```python
from build123d import *

# Parameters (mm, degrees)
F0_W      = 10
F0_H      = 30
F0_R      = 2.125
F1_DEPTH  = 5
F2_W      = 10
F2_H      = 30
F3_DEPTH  = 4
F4_W      = 10
F4_H      = 14.15
F5_DEPTH  = 20
F7_DEPTH  = 10.001
F8_R      = 2.125
F9_DEPTH  = 22.076
F11_DEPTH = 4


with BuildPart() as f1:
    # F0 (on Top) → F1 (new body)
    with BuildSketch(Plane.XY):
        Rectangle(F0_W, F0_H)
        with Locations((1, -10)):
            Circle(F0_R, mode=Mode.SUBTRACT)
        with Locations((1, 10)):
            Circle(F0_R, mode=Mode.SUBTRACT)
    extrude(amount=F1_DEPTH)

    # F2 (on face) → F3 (join)
    with BuildSketch(Plane.XY.offset(5)):
        Rectangle(F2_W, F2_H)
        Polygon((-0.68875, -7.075), (2.68875, -7.075), (4.377499, -10), (2.68875, -12.925), (-0.68875, -12.925), (-2.377499, -10), align=None, mode=Mode.SUBTRACT)
        Polygon((4.377499, 10), (2.68875, 7.075), (-0.68875, 7.075), (-2.377499, 10), (-0.68875, 12.925), (2.68875, 12.925), align=None, mode=Mode.SUBTRACT)
    extrude(amount=F3_DEPTH)

    # F4 (on face) → F5 (join)
    with BuildSketch(Plane.XY.offset(9)):
        Rectangle(F4_W, F4_H)
    extrude(amount=F5_DEPTH)

    # F6 (on face) → F7 (cut, through all)
    with BuildSketch(Plane.YZ.offset(5)):
        with BuildLine():
            ThreePointArc((-3, 12.139388), (0, 5), (3, 12.139388))
            Line((3, 12.139388), (3, 29))
            Line((3, 29), (-3, 29))
            Line((-3, 29), (-3, 12.139388))
        make_face()
    extrude(amount=-F7_DEPTH, mode=Mode.SUBTRACT)

    # F8 (on face) → F9 (cut, through all)
    with BuildSketch(Plane.XZ.offset(7.075)):
        with Locations((0, 21.5)):
            Circle(F8_R)
    extrude(amount=-F9_DEPTH, mode=Mode.SUBTRACT)

    # F10 (on face) → F11 (join)
    with BuildSketch(Plane(origin=(0, 7.075, 0), x_dir=(-1, 0, 0), z_dir=(0, 1, 0))):
        Polygon((5, 18.613249), (5, 24.386751), (0, 27.273503), (-5, 24.386751), (-5, 18.613249), (0, 15.726497), align=None)
        Polygon((0, 24.877499), (2.925, 23.18875), (2.925, 19.81125), (0, 18.122501), (-2.925, 19.81125), (-2.925, 23.18875), align=None, mode=Mode.SUBTRACT)
    extrude(amount=F11_DEPTH)


solid = f1.part
```
Verification items for the finished model (mm, model axes). A direction names the side the tool comes from. Coordinates: 2 decimals unless noted, no trailing zeros. Loops run counter-clockwise (first coordinate to the right, second up) from the corner with the lowest first, then second, coordinate; pieces in that order, holes last. Notation, with made-up numbers: (-14, 64.25) -> (31, 64.25) arc R28 cw to (31, 100.25) -> close; hole circle Ø4 at (37.5, -32.5). An arc over 180 degrees is marked (long way). Answer in a Markdown table with one row per item.
1) Draft check along Y on faces 5 (the face through (-1.521, -11.483, 6.972)), 6 (the face through (0, 7.075, 24)), 7 (the face through (-1, 13, 9)), 8 (the face through (-1.521, 8.517, 6.972)). Enter one of: released by +Y, released by -Y, zero draft, split by the parting line, or undercut.
The answers:
| item | result |
|---|---|
| face 5 | undercut |
| face 6 | released by +Y |
| face 7 | zero draft |
| face 8 | undercut |
2) Section check D-D (y = -7.5). Record the cut outline in (x, z).
The answers:
| item | result |
|---|---|
| outline | (-5, 0) -> (5, 0) -> (5, 9) -> (2.93, 9) -> (2.93, 5) -> (-0.93, 5) -> (-0.93, 9) -> (-5, 9) -> close |
3) Section check C-C (x = 1). Give the number of separate pieces and of enclosed holes in the cut face, and give its area (3 significant figures).
The answers:
| item | result |
|---|---|
| separate pieces | 5 |
| enclosed holes | 0 |
| area | 301 mm2 |
4) Section check A-A (z = 21.5). Record the cut outline in (x, y) (3 decimals).
The answers:
| item | result |
|---|---|
| outline | (-5, -7.075) -> (-2.125, -7.075) -> (-2.125, -3) -> (-5, -3) -> close; (-5, 3) -> (-2.125, 3) -> (-2.125, 7.075) -> (-2.925, 7.075) -> (-2.925, 11.075) -> (-5, 11.075) -> close; (2.125, -7.075) -> (5, -7.075) -> (5, -3) -> (2.125, -3) -> close; (2.125, 3) -> (5, 3) -> (5, 11.075) -> (2.925, 11.075) -> (2.925, 7.075) -> (2.125, 7.075) -> close |
5) Section check B-B (y = 9). Record the cut outline in (x, z) (1 decimal).
The answers:
| item | result |
|---|---|
| outline | (-5, 0) -> (-0.9, 0) -> (-0.9, 5) -> (-1.8, 5) -> (-1.8, 9) -> (-5, 9) -> close; (-5, 18.6) -> (0, 15.7) -> (5, 18.6) -> (5, 24.4) -> (0, 27.3) -> (-5, 24.4) -> close; (2.9, 0) -> (5, 0) -> (5, 9) -> (3.8, 9) -> (3.8, 5) -> (2.9, 5) -> close; hole (-2.9, 19.8) -> (0, 18.1) -> (2.9, 19.8) -> (2.9, 23.2) -> (0, 24.9) -> (-2.9, 23.2) -> close |
6) Access from +Z, -Z, +X, -X, +Y, -Y to the whole of each face (thin tool, end or side, straight path). Record for faces 1 (the face through (3.2, -9.3, 5)), 2 (the face through (2.535, 9.047, 17.19)), 3 (the face through (1.442, 9.047, 18.955)), 4 (the face through (0, 3, 19)).
The answers:
| item | result |
|---|---|
| face 1 | +Z |
| face 2 | +X, +Y |
| face 3 | +Y |
| face 4 | +Z, +X, -X |
7) Depth check by flat-ended pin: P1, Ø5.5, axis at x = 1, y = -10, coming from the +Z side; P2, Ø1.5, axis at x = -4, z = 25.5, coming from the -Y side (3 decimals); P3, Ø2, axis at x = 2, z = 11, coming from the +Y side (3 decimals); P4, Ø1.5, axis at x = -1, y = -2.5, coming from the +Z side. Enter the tip coordinate at first touch or a pass-through.
The answers:
| item | result |
|---|---|
| P1 | stops at z = 5 |
| P2 | stops at y = -7.075 |
| P3 | stops at y = 7.075 |
| P4 | stops at z = 29 |
8) Scan lines: line 1 along Y through (x, z) = (1, 2.95) (3 decimals); line 2 along Y through (x, z) = (3.5, 23.25) (3 decimals); line 3 along Z through (x, y) = (2.75, 8.75). Record each from-to range of solid material in increasing order. Write a range as from..to.
The answers:
| item | result |
|---|---|
| line 1 | y = -15..-12.125, -7.875..7.875, 12.125..15 |
| line 2 | y = -7.075..-3, 3..11.075 |
| line 3 | z = 0..5, 17.31..19.71, 23.29..25.69 |
